The listing builds one solid part. Answer for the finished solid, in the listing's coordinates (mm). Coordinates: 2 decimals unless noted, no trailing zeros. Order: outer loops, then holes, each group sorted by start corner. A loop starts at its lowest first (then second) coordinate and runs counter-clockwise, first axis right, second up. Notation, with made-up numbers: (47, -38.5) -> (57, -38.5) arc R23 cw to (57, -6.5) -> close; hole circle Ø10 at (44.25, 84). An arc over 180 degrees is marked (long way). Write each question's results on one line, items separated by ' | '. Start each with the question number.
(1) Given pin 1 (4.5 mm diameter, centred on x = 74.5, z = 14, fed in from -Y); pin 2 (4.5 mm diameter, centred on x = 71, z = 5.5, fed in from +Y); pin 3 (8 mm diameter, centred on x = 78.82, y = 3, fed in from +Z), each flat-ended and moving along its own axis, determine where each tip first touches the part or whether it passes through.
(2) The part is cut by section A-A, the plane z = 10.5. Give the vertices of the cut face in (x, y).
(3) The part is cut by section B-B, the plane y = 3. Count the separate pieces of the cut face and the enclosed holes in it, then the cut area to 3 significant figures.
(4) Straight lines are drawn through the part: L1, parallel to Z at x = 73, y = 0.5; L2, parallel to X at y = 1.75, z = 4.25; L3, parallel to X at y = 0.25, z = 9.5. For each, find the intervals that lie inside material, in ascending order.
(5) The part is cut by section C-C, the plane x = 40.5. Give the vertices of the cut face in (y, z).
(6) The part is cut by section D-D, the plane x = -20. Give the vertices of the cut face in (y, z), then the cut area to 3 significant figures.
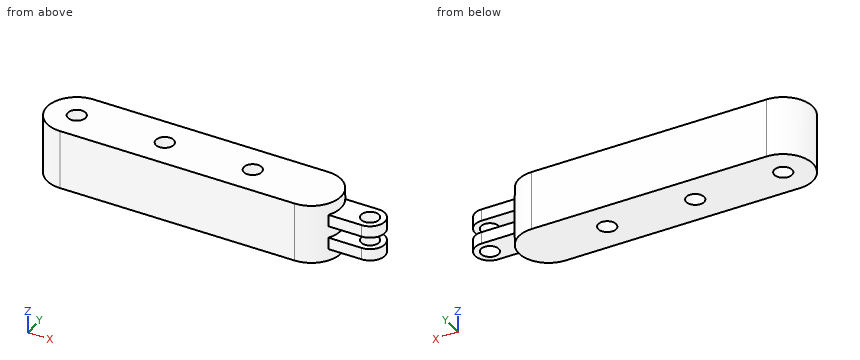
Autodesk Inventor part; units mm, degrees
ref_plane "Work Plane5" through (0, 0, 12) normal (0, 0, 1) x (1, 0, 0)
ref_plane "Work Plane6" through (0, 0, 10) normal (0, 0, 1) x (1, 0, 0)
ref_plane "YZ Plane" through (0, 0, 0) normal (1, 0, 0) x (0, 1, 0)
sketch "Sketch1" plane through (0, 0, 0) normal (0, 0, 1) x (1, 0, 0)
  line L0 (-21.1783, 3) -> (58.8217, 3) construction
  line L1 (-21.1783, -7) -> (58.8217, -7)
  line L2 (58.8217, 13) -> (-21.1783, 13)
  arc A0 (-21.1783, 13) -> (-21.1783, -7) centre (-21.1783, 3) ccw
  arc A1 (58.8217, -7) -> (58.8217, 13) centre (58.8217, 3) ccw
  line L3 (67.482, 8) -> (78.8217, 8)
  arc A2 (78.8217, -2) -> (78.8217, 8) centre (78.8217, 3) ccw
  line L4 (67.482, -2) -> (78.8217, -2)
  circle A3 centre (78.8217, 3) radius 3
  circle A4 centre (8.8217, 3) radius 3
  circle A5 centre (38.8217, 3) radius 3
  circle A6 centre (-21.1783, 3) radius 3
  point P0 (0, 0)
  dimension "d0" = 20
  dimension "d18" = 10
  dimension "d19" = 20
  dimension "d21" = 6
  dimension "d29" = 30
  dimension "d31" = 30
extrude "Extrusion1" add sketch "Sketch1" along normal blind 20 contours A0 L2 A1 L1
ref_plane "Work Plane5" through (0, 0, 12) normal (0, 0, 1) x (1, 0, 0)
ref_plane "Work Plane4" through (0, 0, 10) normal (0, 0, 1) x (1, 0, 0)
sketch "Sketch4" plane through (0, 0, 12) normal (0, 0, 1) x (1, 0, 0)
  line L0 (67.482, 8) -> (78.8217, 8)
  line L1 (67.482, -2) -> (78.8217, -2)
  arc A0 (78.8217, -2) -> (78.8217, 8) centre (78.8217, 3) ccw
  circle A1 centre (78.8217, 3) radius 3
  arc A2 (58.8217, -7) -> (58.8217, 13) centre (58.8217, 3) ccw
  point P0 (0, 0)
extrude "Extrusion4" add sketch "Sketch4" along normal blind 4
ref_plane "Work Plane6" through (0, 0, 10) normal (0, 0, 1) x (1, 0, 0)
mirror "Mirror2" about plane through (0, 0, 10) normal (0, 0, 1) of "Extrusion4"
equation "\"d18\" = R"
equation "\"d21\" = r"
equation "\"d6\" = w"
equation "\"d22\" = 0.2 * w"
equation "\"r\" = 6"
equation "\"d3\" = 6"
equation "\"d5\" = 6"
equation "\"th\" = 5"
equation "\"R\" = 10"
equation "\"w\" = 20"
equation "\"d20\" = 0.1 * w"
equation "\"d25\" = 6"
Established:
1) pin 1: stops at y = -2 | pin 2: stops at y = 8 | pin 3: stops at z = 16
2) outline: (-21.18, -7) -> (58.82, -7) arc R10 ccw to (58.82, 13) -> (-21.18, 13) arc R10 ccw to start; hole circle Ø6 at (-21.18, 3); hole circle Ø6 at (8.82, 3); hole circle Ø6 at (38.82, 3)
3) separate pieces: 6 | enclosed holes: 0 | area: 1,710 mm^2
4) L1: z = 4 to 8, 12 to 16 | L2: x = -31.1 to -23.91, -18.45 to 6.09, 11.55 to 36.09, 41.55 to 76.09, 81.55 to 83.66 | L3: x = -30.79 to -22.38, -19.98 to 7.62, 10.02 to 37.62, 40.02 to 68.44
5) outline: (-7, 0) -> (0.51, 0) -> (0.51, 20) -> (-7, 20) -> close; (5.49, 0) -> (13, 0) -> (13, 20) -> (5.49, 20) -> close
6) outline: (-7, 0) -> (0.24, 0) -> (0.24, 20) -> (-7, 20) -> close; (5.76, 0) -> (13, 0) -> (13, 20) -> (5.76, 20) -> close | area: 290 mm^2
